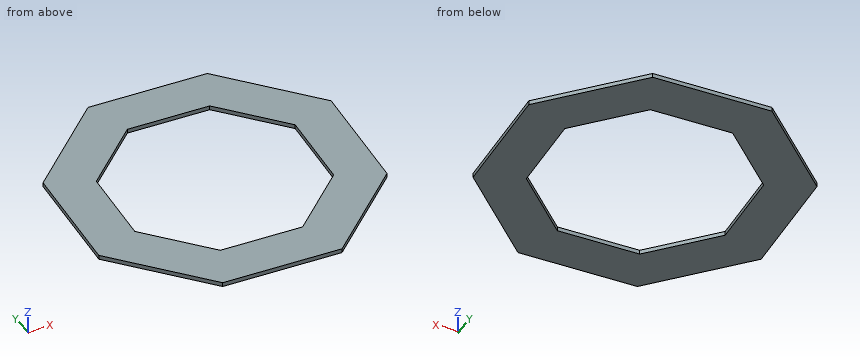
```python
from build123d import *

# Parameters (mm, degrees)
SALIENTE_EXTRUIR1_DEPTH = 3
CORTAR_EXTRUIR1_DEPTH   = 3


with BuildPart() as part:
    # Croquis1 → Saliente-Extruir1 (new body)
    with BuildSketch(Plane.XY):
        Polygon((-45.692015403, -98.122211965), (37.073747528, -101.692015403), (98.122211965, -45.692015403), (101.692015403, 37.073747528), (45.692015403, 98.122211965), (-37.073747528, 101.692015403), (-98.122211965, 45.692015403), (-101.692015403, -37.073747528), align=None)
    extrude(amount=SALIENTE_EXTRUIR1_DEPTH)

    # Croquis2 → Cortar-Extruir1 (cut)
    with BuildSketch(Plane(origin=(0, 0, 0), x_dir=(-1, 0, 0), z_dir=(0, 0, -1))):
        Polygon((-67.704326256, -31.527490628), (-25.580885794, -70.167490628), (31.527490628, -67.704326256), (70.167490628, -25.580885794), (67.704326256, 31.527490628), (25.580885794, 70.167490628), (-31.527490628, 67.704326256), (-70.167490628, 25.580885794), align=None)
    extrude(amount=-CORTAR_EXTRUIR1_DEPTH, mode=Mode.SUBTRACT)


solid = part.part
```
Geometry check sheet. Reference: the model listing, model coordinates, mm. Give positions to 0.01 mm unless a question says otherwise; leave off trailing zeros. Loops run counter-clockwise (first coordinate to the right, second up) from the corner with the lowest first, then second, coordinate; pieces in that order, holes last. Notation, with made-up numbers: M 28.5,73.25 L 76.5,73.25 A16 ccw 76.5,99.25 Z; hole C 29,-25.75 d8. An arc over 180 degrees is marked long. Write item = value, one per line.
(1) Sectioned sample at A-A, the plane z = 0.5. Record the cut outline in (x, y), plus the area to 3 significant figures.
Answer below:
outline = M -101.69,-37.07 L -45.69,-98.12 L 37.07,-101.69 L 98.12,-45.69 L 101.69,37.07 L 45.69,98.12 L -37.07,101.69 L -98.12,45.69 Z; hole M -70.17,-25.58 L -31.53,-67.7 L 25.58,-70.17 L 67.7,-31.53 L 70.17,25.58 L 31.53,67.7 L -25.58,70.17 L -67.7,31.53 Z
area = 17,400 mm2
(2) Gauge pin test, flat ends, axial feed: pin 1 Ø5 at (x, y) = (19.5, -66.5) entering from +Z; pin 2 Ø1.5 at (y, z) = (-16.5, 2.5) entering from +X. Record the tip position at first contact, or that the pin passes through.
Answer below:
pin_1 = through
pin_2 = 99.41
(3) Sectioned sample at B-B, the plane x = -16. Record the cut outline in (y, z), plus the area to 3 significant figures.
Answer below:
outline = M -99.4,0 L -68.37,0 L -68.37,3 L -99.4,3 Z; M 69.75,0 L 100.78,0 L 100.78,3 L 69.75,3 Z
area = 186 mm2
(4) Sectioned sample at D-D, the plane x = -78. Record the cut outline in (y, z), plus the area to 3 significant figures.
Answer below:
outline = M -62.9,0 L 64.15,0 L 64.15,3 L -62.9,3 Z
area = 381 mm2
(5) Sectioned sample at C-C, the plane y = 12.5. Record the cut outline in (x, z) (3 decimals).
Answer below:
outline = M -99.554,0 L -68.525,0 L -68.525,3 L -99.554,3 Z; M 69.603,0 L 100.632,0 L 100.632,3 L 69.603,3 Z
(6) Material ranges on line 1 (Y direction, x = -10, z = 0.65); line 2 (X direction, y = -65.5, z = 0.45); line 3 (Y direction, x = -44, z = 1.95), recorded low to high. Write a range as [from, to].
Answer below:
line_1 = [-99.66, -68.63], [69.5, 100.52]
line_2 = [-75.62, -33.55], [30.67, 76.53]
line_3 = [-98.2, -54.11], [53.27, 95.34]
